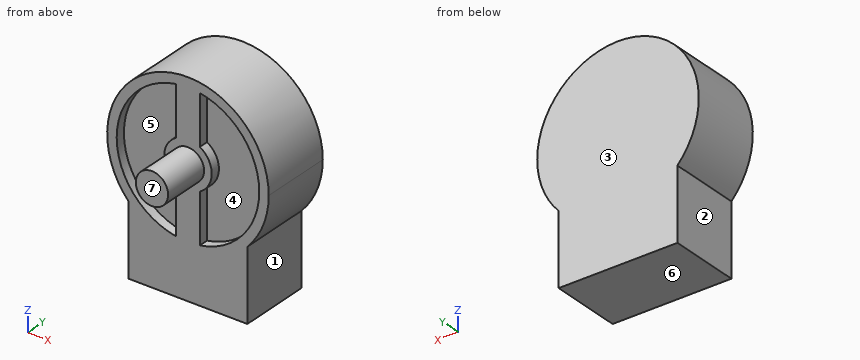
```python
from build123d import *

# Parameters (mm, degrees)
F1_DEPTH = 15
F3_DEPTH = 2
F4_R     = 3.4
F5_DEPTH = 10


# Not quite as in the source:
# - a feature of the source that left no trace in its solid (it failed there, or was rolled back) is left out
# - a pattern or mirror of a feature is missing from the dataset's text; its kind, count and spacing are read off the source's solid


with BuildPart() as f1:
    # F0 (on Front) → F1 (new body)
    with BuildSketch(Plane.XZ):
        with BuildLine():
            ThreePointArc((12.5, -11.5217186218), (15.8350876221, -6.1846584384), (17, 0))
            ThreePointArc((17, 0), (-6.1846584384, 15.8350876221), (-12.5, -11.5217186218))
            ThreePointArc((-12.5, -11.5217186218), (0, -17), (12.5, -11.5217186218))
        make_face()
        with BuildLine():
            ThreePointArc((12.5, -11.5217186218), (0, -17), (-12.5, -11.5217186218))
            Line((-12.5, -11.5217186218), (-12.5, -26.5217186218))
            Line((-12.5, -26.5217186218), (12.5, -26.5217186218))
            Line((12.5, -26.5217186218), (12.5, -11.5217186218))
        make_face()
    extrude(amount=F1_DEPTH)

    # F2 (on face) → F3 (cut)
    with BuildSketch(Plane.XZ.offset(15)):
        with BuildLine():
            Line((-2.5, 4.3301270189), (-2.5, 14.7901994577))
            ThreePointArc((-2.5, 14.7901994577), (-15, 0), (-2.5, -14.7901994577))
            Line((-2.5, -14.7901994577), (-2.5, -4.3301270189))
            ThreePointArc((-2.5, -4.3301270189), (-5, 0), (-2.5, 4.3301270189))
        make_face()
    f3 = extrude(amount=-F3_DEPTH, mode=Mode.SUBTRACT)

    # F3_copies: F3 across plane
    add(f3.mirror(Plane(origin=(0, 0, 0), x_dir=(0, 0, 1), z_dir=(1, 0, 0))), mode=Mode.SUBTRACT)

    # F4 (on face) → F5 (join)
    with BuildSketch(Plane.XZ.offset(15)):
        Circle(F4_R)
    extrude(amount=F5_DEPTH)


solid = f1.part
```
Model file for the job. Use its own axes, mm. Face numbers are marked on the shaded views. A direction names the side the tool comes from. Round coordinates to 2 decimals unless told otherwise and drop trailing zeros. Write each loop counter-clockwise with the first axis right and the second up, starting at its lowest first coordinate (ties: lowest second). Pieces come first, ordered by that corner, then holes. Notation, with made-up numbers: (3, 12.5) - (36, 12.5) arc R21 ccw to (36, 18.5) - close; hole circle Ø1 at (-18, 23). An arc over 180 degrees is marked (long way). One line per item, written item: value.
(1) Cut at C-C, the plane y = -5. Give the cut face in (x, z).
Values follow:
outline: (-12.5, -26.52) - (12.5, -26.52) - (12.5, -11.52) arc R17 ccw (long way) to (-12.5, -11.52) - close
(2) Cut at A-A, the plane y = -14.5. Give the cut face in (x, z).
Values follow:
outline: (-12.5, -26.52) - (12.5, -26.52) - (12.5, -11.52) arc R17 ccw (long way) to (-12.5, -11.52) - close; hole (-2.5, -14.79) - (-2.5, -4.33) arc R5 cw to (-2.5, 4.33) - (-2.5, 14.79) arc R15 ccw to start; hole (2.5, -14.79) arc R15 ccw to (2.5, 14.79) - (2.5, 4.33) arc R5 cw to (2.5, -4.33) - close
(3) Cut at B-B, the plane x = 0. Give the cut face in (y, z), plus the area to 3 significant figures.
Values follow:
outline: (-25, -3.4) - (-15, -3.4) - (-15, -26.52) - (0, -26.52) - (0, 17) - (-15, 17) - (-15, 3.4) - (-25, 3.4) - close
area: 721 mm²
(4) 3-axis set-ups, long thin cutter, end or side, ignore diameter. For the marked faces 1, 2, 3 and 4: which of +Z, -Z, +X, -X, +Y, -Y reach the whole face in a straight line?
Values follow:
face 1: -Z, +X, +Y, -Y
face 2: -Z, -X, +Y, -Y
face 3: +Z, -Z, +X, -X, +Y
face 4: -Y
(5) Drop flat-ended pins along their axis: P1, Ø5, axis at y = -15, z = 11.5, coming from the +X side; P2, Ø1, axis at y = -13.5, z = -7, coming from the +X side; P3, Ø12, axis at y = -8, z = -20.5, coming from the -X side; P4, Ø1.5, axis at x = -10, z = 4, coming from the +Y side. Give the stop position or say it passes through.
Values follow:
P1: stops at x = 14.42
P2: stops at x = 15.71
P3: stops at x = -12.5
P4: stops at y = 0
(6) Cut at D-D, the plane z = 9.5. Give the cut face in (x, y).
Values follow:
outline: (-14.1, -15) - (-11.61, -15) - (-11.61, -13) - (-2.5, -13) - (-2.5, -15) - (2.5, -15) - (2.5, -13) - (11.61, -13) - (11.61, -15) - (14.1, -15) - (14.1, 0) - (-14.1, 0) - close
(7) Two-plate mould, pull along Z, no slides. Class the marked faces 5, 6 and 7: pulls with the +Z half, pulls with the -Z half, needs draft (parallel to the pull), parting line crosses it, or undercut.
Values follow:
face 5: undercut
face 6: pulls with the -Z half
face 7: needs draft
(8) Wall check: probe 1 along X at (y, z) = (-13.75, -11.5); probe 2 along Y at (x, z) = (-8.5, 0); probe 3 along Y at (x, z) = (12.5, 8.5). Give the ranges that are in metal, low to high.
Values follow:
probe 1: x = -12.52 to -9.63, -2.5 to 2.5, 9.63 to 12.52
probe 2: y = -13 to 0
probe 3: y = -15 to 0
